```python
from build123d import *

# Parameters (mm, degrees)
BOSS_EXTRUDE1_DEPTH     = 33.5
CUT_EXTRUDE1_DEPTH      = 50.262054362
CUT_EXTRUDE1_DEPTH_BACK = 50.262054362
SKETCH3_W               = 37.712944555
SKETCH3_H               = 32.806463902
SKETCH4_R               = 2
CUT_EXTRUDE2_DEPTH      = 50.262054362
FILLET1_R               = 2


with BuildPart() as part:
    # Sketch1 → Boss-Extrude1 (new, symmetric)
    with BuildSketch(Plane(origin=(0, 0, 0), x_dir=(1, 0, 0), z_dir=(0, 1, 0))):
        with BuildLine():
            Line((4.849945859, -1.215740583), (1.202724111, -15.76557816))
            Line((1.202724111, -15.76557816), (-17.808565296, -11))
            Line((-17.808565296, -11), (-33.5, -11))
            Line((-33.5, -11), (-33.5, -8.5))
            Line((-33.5, -8.5), (-17.5, -8.5))
            Line((-17.5, -8.5), (-0.614378527, -12.732734939))
            Line((-0.614378527, -12.732734939), (2.42497293, -0.607870291))
            ThreePointArc((2.42497293, -0.607870291), (-1.76517118, 1.77035892), (0.600751286, -2.426746359))
            Line((0.600751286, -2.426746359), (-0.044239613, -4.999804282))
            ThreePointArc((-0.044239613, -4.999804282), (-3.058347209, 3.95556726), (4.849945859, -1.215740583))
        make_face()
    extrude(amount=BOSS_EXTRUDE1_DEPTH, both=True)

    # Sketch3 → Cut-Extrude1 (cut, two sides: drawn at the far end of the back side and taken through both)
    with BuildSketch(Plane(origin=(0, 0, 8.5), x_dir=(-1, 0, 0), z_dir=(0, 0, -1)).offset(-CUT_EXTRUDE1_DEPTH_BACK)):
        with Locations((-1.356472277, 34.403231951)):
            Rectangle(SKETCH3_W, SKETCH3_H)
        with Locations((-1.356472277, -34.403231951)):
            Rectangle(SKETCH3_W, SKETCH3_H)
    extrude(amount=CUT_EXTRUDE1_DEPTH + CUT_EXTRUDE1_DEPTH_BACK, mode=Mode.SUBTRACT)

    # Sketch4 → Cut-Extrude2 (cut, through all)
    with BuildSketch(Plane(origin=(0, 0, 8.5), x_dir=(-1, 0, 0), z_dir=(0, 0, -1))):
        with Locations((25.5, 26.5)):
            Circle(SKETCH4_R)
        with Locations((25.5, -26.5)):
            Circle(SKETCH4_R)
    extrude(amount=-CUT_EXTRUDE2_DEPTH, mode=Mode.SUBTRACT)

    # Fillet1
    fillet1_edges = [part.edges().sort_by_distance(p)[0] for p in [
        (-17.5, -33.5, 9.788674179),
        (-33.5, -33.5, 9.75),
        (-33.5, 33.5, 9.75),
        (-17.5, 33.5, 9.788674179),
    ]]
    fillet(fillet1_edges, radius=FILLET1_R)


solid = part.part
```
The listing builds one solid part. Answer for the finished solid, in the listing's coordinates (mm). A direction names the side the tool comes from. Give positions to 0.01 mm unless a question says otherwise; leave off trailing zeros. Loops run counter-clockwise (first coordinate to the right, second up) from the corner with the lowest first, then second, coordinate; pieces in that order, holes last. Notation, with made-up numbers: (-27.75, 37) - (-11.75, 37) arc R13 cw to (-11.75, 59) - close; hole circle Ø1 at (-6, 1). An arc over 180 degrees is marked (long way). Return JSON: item names as keys, results as strings. Group by question number.
1. Which of the six approach directions +Z, -Z, +X, -X, +Y, -Y give full straight-line access (tool end or side, diameter ignored) to faces 1 (the flat face through (-9.175, 0.252, 10.587)), 2 (the flat face through (-26, 0, 11)), 3 (the flat face through (-1.2, -18, 4.66)), 4 (the flat face through (3.05, 0.25, 8.39)), 5 (the flat face through (-17.5, 25, 10))?
2. Find section D-D (z = -0.5). Write down the section's boundary in (x, y), then the cut area to 3 significant figures.
3. Straight lines are drawn through the part: line 1 (Y direction, x = -25.5, z = 10); line 2 (X direction, y = -5.5, z = 0); line 3 (X direction, y = -8, z = 1.75). For each, find the intervals that lie inside material, in ascending order. Write a range as [from, to].
4. Find section B-B (y = 6). Write down the section's boundary in (x, z).
5. Find section A-A (x = -25.5). Write down the section's boundary in (y, z).
6. Determine the mould class of faces 6 (the cylindrical face through (-32.9, -32.93, 9.73)), 7 (the cylindrical face through (-23.9, -27.7, 9.7)), 8 (the flat face through (-25, -33.5, 10)), 9 (the cylindrical face through (-25.066, 24.548, 9.732)) for opening direction X: pulls with the +X half, pulls with the -X half, needs draft (parallel to the pull), parting line crosses it, or undercut.
7. Given pin 1 Ø6 at (y, z) = (12, 3.5) entering from +X; pin 2 Ø1 at (y, z) = (-13, 2.5) entering from +X; pin 3 Ø8 at (y, z) = (10.5, 13.5) entering from +X; pin 4 Ø12 at (x, z) = (-18.5, 3.5) entering from -Y, each flat-ended and moving along its own axis, determine where each tip first touches the part or whether it passes through.
8. Find section C-C (y = -26.5). Write down the section's boundary in (x, z), then the cut area to 3 significant figures.
Verdict:
{
 "1": {"face 1": "+Y, -Y", "face 2": "+Z, -X, +Y, -Y", "face 3": "+Z, -Z, +X, -Y", "face 4": "+Z, +X, +Y, -Y", "face 5": "+Z, -Z, +X, +Y"},
 "2": {"outline": "(-4.97, -18) - (-2.45, -18) - (-2.45, 18) - (-4.97, 18) - close; (2.45, -18) - (4.97, -18) - (4.97, 18) - (2.45, 18) - close", "area": "182 mm^2"},
 "3": {"line 1": "y = [-33.5, -28.5], [-24.5, 24.5], [28.5, 33.5]", "line 2": "x = [-5, -2.5], [2.5, 5]", "line 3": "x = [-4.68, -1.79], [2.14, 4.72]"},
 "4": {"outline": "(-33.5, 8.5) - (-17.5, 8.5) - (-0.61, 12.73) - (2.42, 0.61) arc R2.5 cw (long way) to (0.6, 2.43) - (-0.04, 5) arc R5 ccw (long way) to (4.85, 1.22) - (1.2, 15.77) - (-17.81, 11) - (-33.5, 11) - close"},
 "5": {"outline": "(-33.5, 8.5) - (-28.5, 8.5) - (-28.5, 11) - (-33.5, 11) - close; (-24.5, 8.5) - (24.5, 8.5) - (24.5, 11) - (-24.5, 11) - close; (28.5, 8.5) - (33.5, 8.5) - (33.5, 11) - (28.5, 11) - close"},
 "6": {"face 6": "pulls with the -X half", "face 7": "undercut", "face 8": "needs draft", "face 9": "undercut"},
 "7": {"pin 1": "stops at x = 4.97", "pin 2": "stops at x = 4.65", "pin 3": "stops at x = 2.77", "pin 4": "stops at y = -33.5"},
 "8": {"outline": "(-33.5, 8.5) - (-27.5, 8.5) - (-27.5, 11) - (-33.5, 11) - close; (-23.5, 8.5) - (-17.5, 8.5) - (-17.5, 11.08) - (-17.81, 11) - (-23.5, 11) - close", "area": "30.0 mm^2"}
}
